CAD build for the part. Positions are in the model's coordinates, mm. A direction names the side the tool comes from. Round coordinates to 2 decimals unless told otherwise and drop trailing zeros.
Solid Edge part; units mm, degrees
sketch "Sketch1" plane through (0, 0, 0) normal (0, 0, 1) x (1, 0, 0)
  line L0 (0, 0) -> (400, 0)
  line L1 (400, 0) -> (400, 100)
  line L2 (400, 100) -> (0, 100)
  line L3 (0, 100) -> (0, 0)
  dimension "D1" = 400
extrude "Protrusion1" add sketch "Sketch1" against normal blind 30
hole "Hole_1" at (50, 80, 0) direction (0, 0, -1) diameter 8.376 depth 25 tip angle 118 thread major 10 thread length 20
hole "Hole1" at (50, 20, 0) direction (0, 0, -1) diameter 8.376 depth 25 tip angle 118 thread major 10 thread length 20
hole "Hole2" at (110, 80, 0) direction (0, 0, -1) diameter 8.376 depth 25 tip angle 118 thread major 10 thread length 20
hole "Hole3" at (110, 20, 0) direction (0, 0, -1) diameter 8.376 depth 25 tip angle 118 thread major 10 thread length 20
hole "Hole4" at (170, 80, 0) direction (0, 0, -1) diameter 8.376 depth 25 tip angle 118 thread major 10 thread length 20
hole "Hole5" at (230, 80, 0) direction (0, 0, -1) diameter 8.376 depth 25 tip angle 118 thread major 10 thread length 20
hole "Hole6" at (170, 20, 0) direction (0, 0, -1) diameter 8.376 depth 25 tip angle 118 thread major 10 thread length 20
hole "Hole7" at (230, 20, 0) direction (0, 0, -1) diameter 8.376 depth 25 tip angle 118 thread major 10 thread length 20
hole "Hole8" at (290, 80, 0) direction (0, 0, -1) diameter 8.376 depth 25 tip angle 118 thread major 10 thread length 20
hole "Hole9" at (350, 80, 0) direction (0, 0, -1) diameter 8.376 depth 25 tip angle 118 thread major 10 thread length 20
hole "Hole10" at (290, 20, 0) direction (0, 0, -1) diameter 8.376 depth 25 tip angle 118 thread major 10 thread length 20
hole "Hole11" at (350, 20, 0) direction (0, 0, -1) diameter 8.376 depth 25 tip angle 118 thread major 10 thread length 20
Item 1: 3-axis set-ups, long thin cutter, end or side, ignore diameter. For faces 1 (the cylindrical face through (345.85, 80.55, -12.68)), 2 (the flat face through (197, 51, 0)): which of +Z, -Z, +X, -X, +Y, -Y reach the whole face in a straight line?
Answers follow:
face 1: +Z
face 2: +Z, +X, -X, +Y, -Y
Item 2: Cut at A-A, the plane z = -5.5. State how many separate pieces and enclosed holes the cut face has, plus the area to 3 significant figures.
Answers follow:
separate pieces: 1
enclosed holes: 12
area: 39,300 mm2
Item 3: Two-plate mould, pull along X, no slides. Class faces 3 (the flat face through (400, 49, -15)), 4 (the conical face through (109.29, 20.16, -27.08)), 5 (the flat face through (203, 100, -15)): released by +X, released by -X, zero draft, split by the parting line, or undercut.
Answers follow:
face 3: released by +X
face 4: undercut
face 5: zero draft
Item 4: Probe line 1 (Y direction, x = 230, z = -17); line 2 (Y direction, x = 48, z = -11). List the from-to ranges inside material, lowest first.
Answers follow:
line 1: y = 0 to 15.81, 24.19 to 75.81, 84.19 to 100
line 2: y = 0 to 16.32, 23.68 to 76.32, 83.68 to 100
Item 5: Flat gauge pins, fed straight in: P1, Ø7.5, axis at x = 170, y = 80, coming from the +Z side; P2, Ø6.5, axis at x = 110, y = 80, coming from the +Z side. Where does each tip first touch, or does it go through?
Answers follow:
P1: stops at z = -25.26
P2: stops at z = -25.56
